Build history of the part. All positions in model axes, mm. A direction names the side the tool comes from. Round coordinates to 2 decimals unless told otherwise and drop trailing zeros. Write each loop counter-clockwise with the first axis right and the second up, starting at its lowest first coordinate (ties: lowest second). Pieces come first, ordered by that corner, then holes.
from build123d import *

# Parameters (mm, degrees)
F0_W     = 15
F0_H     = 15
F1_DEPTH = 5
F3_DEPTH = 2.5


with BuildPart() as f1:
    # F0 (on Top) → F1 (new body)
    with BuildSketch(Plane.XY):
        Rectangle(F0_W, F0_H)
    extrude(amount=F1_DEPTH)

    # F2 (on face) → F3 (cut)
    with BuildSketch(Plane.XY.offset(5)):
        Polygon((0, 2.502102), (-1.851563, 3.663132), (-4.242188, -0.149336), (-2.25, -1.398546), (-2.25, -3.75), (2.25, -3.75), (2.25, -1.398546), (4.242187, -0.149336), (1.851562, 3.663132), align=None)
    extrude(amount=-F3_DEPTH, mode=Mode.SUBTRACT)


solid = f1.part
1) Which spindle directions (+Z, -Z, +X, -X, +Y, -Y) get a long thin tool onto all of the face, cutting with end or side? Do faces 4 (the flat face through (-2.25, -3, 4)), 5 (the flat face through (7.5, 0, 2)). Say none if no direction does.
Results:
face 4: +Z
face 5: +Z, -Z, +X, +Y, -Y
2) Slice it at B-B (y = -2.5). Write the cut outline in (x, z).
Results:
outline: (-7.5, 0) - (7.5, 0) - (7.5, 5) - (2.25, 5) - (2.25, 2.5) - (-2.25, 2.5) - (-2.25, 5) - (-7.5, 5) - close
3) Slice it at A-A (z = 3.15). Write the cut outline in (x, y).
Results:
outline: (-7.5, -7.5) - (7.5, -7.5) - (7.5, 7.5) - (-7.5, 7.5) - close; hole (-4.24, -0.15) - (-2.25, -1.4) - (-2.25, -3.75) - (2.25, -3.75) - (2.25, -1.4) - (4.24, -0.15) - (1.85, 3.66) - (0, 2.5) - (-1.85, 3.66) - close
4) Wall check: L1, parallel to X at y = -3.5, z = 4.2; L2, parallel to Z at x = -0.75, y = 0.5; L3, parallel to Y at x = -2.5, z = 4.2. Give the ranges that are in metal, low to high.
Results:
L1: x = -7.5 to -2.25, 2.25 to 7.5
L2: z = 0 to 2.5
L3: y = -7.5 to -1.24, 2.63 to 7.5
5) Slice it at D-D (y = 3). Write the cut outline in (x, z).
Results:
outline: (-7.5, 0) - (7.5, 0) - (7.5, 5) - (2.27, 5) - (2.27, 2.5) - (0.79, 2.5) - (0.79, 5) - (-0.79, 5) - (-0.79, 2.5) - (-2.27, 2.5) - (-2.27, 5) - (-7.5, 5) - close
6) Slice it at C-C (x = 3). Write the cut outline in (y, z), plus the area to 3 significant figures.
Results:
outline: (-7.5, 0) - (7.5, 0) - (7.5, 5) - (1.83, 5) - (1.83, 2.5) - (-0.93, 2.5) - (-0.93, 5) - (-7.5, 5) - close
area: 68.1 mm2
7) Mould opens along X. For faces 1 (the flat face through (3.232, -0.783, 3.768)), 2 (the flat face through (0, -7.5, 2)), 3 (the flat face through (-7.5, 0, 2)) say: released by +X, released by -X, zero draft, split by the parting line, or undercut.
Results:
face 1: undercut
face 2: zero draft
face 3: released by -X
